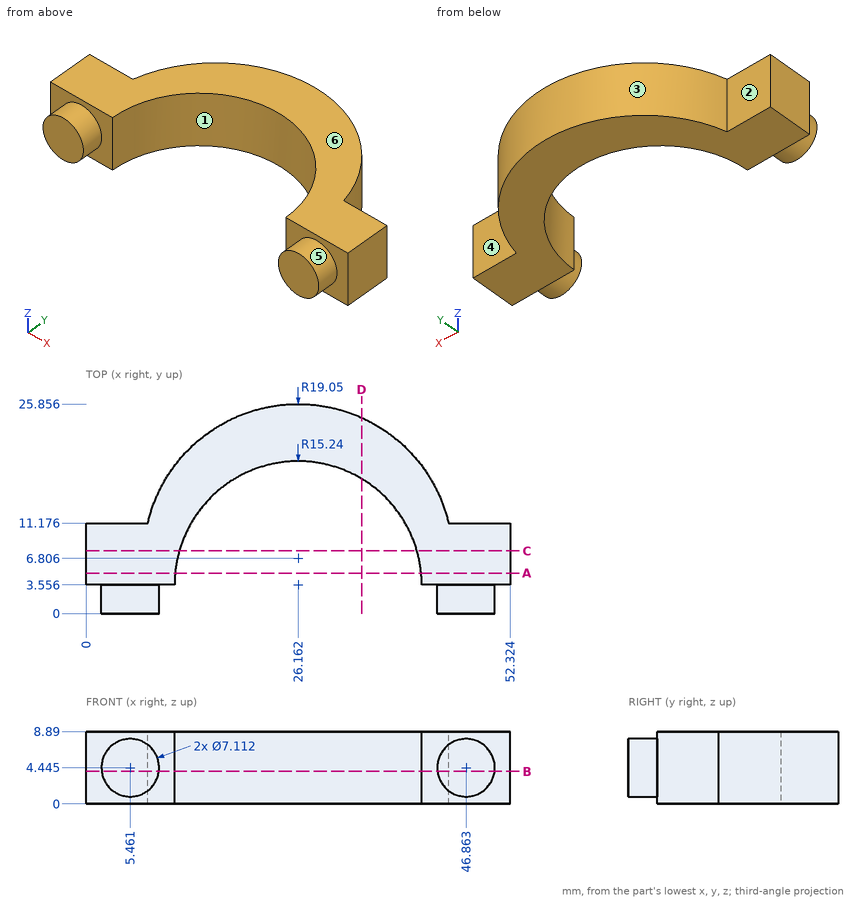
Source: three-view drawing plus pictorial views. Frame: mm from the lowest corner of the part. A direction names the side the tool comes from. Give positions to 0.01 mm unless a question says otherwise; leave off trailing zeros. Loops run counter-clockwise (first coordinate to the right, second up) from the corner with the lowest first, then second, coordinate; pieces in that order, holes last. Notation, with made-up numbers: (-35.75, 3.25) -> (6.25, 3.25) arc R25 ccw to (6.25, 25.25) -> close; hole circle Ø6 at (-6.75, -35). An arc over 180 degrees is marked (long way). Use a Markdown table: item, result. Add a question column.
(1) Section query D-D (x = 34). Output: boundary loops of the cut face in (y, z), then the cut area to 3 significant figures.
(2) Section query C-C (y = 7.75). Output: boundary loops of the cut face in (x, z), then the cut area to 3 significant figures.
(3) Ray query, line 1 (X direction, y = 9, z = 7); line 2 (X direction, y = 12.5, z = 1.25); line 3 (Y direction, x = 5.5, z = 6). Return the intervals inside material, ascending.
(4) Section query B-B (z = 4). Output: boundary loops of the cut face in (x, y) (3 decimals).
(5) Section query A-A (y = 5). Output: boundary loops of the cut face in (x, z), then the cut area to 3 significant figures.
(6) Access query for the marked faces 4, 5 and 6. Directions: +Z, -Z, +X, -X, +Y, -Y. A direction counts if a zero-diameter tool reaches every point of the face in a straight line with its end or side. Return the directions, or none.
(7) First-contact query: pin 1 Ø5 at (y, z) = (6, 7.5) entering from -X; pin 2 Ø4 at (x, z) = (49, 4) entering from +Y. Flat tips, straight axial feed; report the tip coordinate or a pass-through.
(8) Pull-direction query (X, two-part tool) for the marked faces 1, 2 and 3; classes: +X half, -X half, draft (parallel to the pull), parting line (faces both ways), or undercut.
Checked values:
| question | item | result |
|---|---|---|
| 1 | outline | (16.63, 0) -> (24.17, 0) -> (24.17, 8.89) -> (16.63, 8.89) -> close |
| 1 | area | 67.1 mm^2 |
| 2 | outline | (0, 0) -> (11.51, 0) -> (11.51, 8.89) -> (0, 8.89) -> close; (40.81, 0) -> (52.32, 0) -> (52.32, 8.89) -> (40.81, 8.89) -> close |
| 2 | area | 205 mm^2 |
| 3 | line 1 | 0 to 11.93, 40.4 to 52.32 |
| 3 | line 2 | 7.98 to 13.82, 38.5 to 44.34 |
| 3 | line 3 | 0 to 11.18 |
| 4 | outline | (0, 3.556) -> (1.933, 3.556) -> (1.933, 0) -> (8.989, 0) -> (8.989, 3.556) -> (10.922, 3.556) arc R15.24 cw to (41.402, 3.556) -> (43.335, 3.556) -> (43.335, 0) -> (50.391, 0) -> (50.391, 3.556) -> (52.324, 3.556) -> (52.324, 11.176) -> (44.704, 11.176) arc R19.05 ccw to (7.62, 11.176) -> (0, 11.176) -> close |
| 5 | outline | (0, 0) -> (10.99, 0) -> (10.99, 8.89) -> (0, 8.89) -> close; (41.33, 0) -> (52.32, 0) -> (52.32, 8.89) -> (41.33, 8.89) -> close |
| 5 | area | 195 mm^2 |
| 6 | face 4 | +Z, -Z, +X, +Y |
| 6 | face 5 | -Y |
| 6 | face 6 | +Z, +X, -X, +Y, -Y |
| 7 | pin 1 | x = 0 |
| 7 | pin 2 | y = 11.18 |
| 8 | face 1 | undercut |
| 8 | face 2 | draft |
| 8 | face 3 | parting line |
